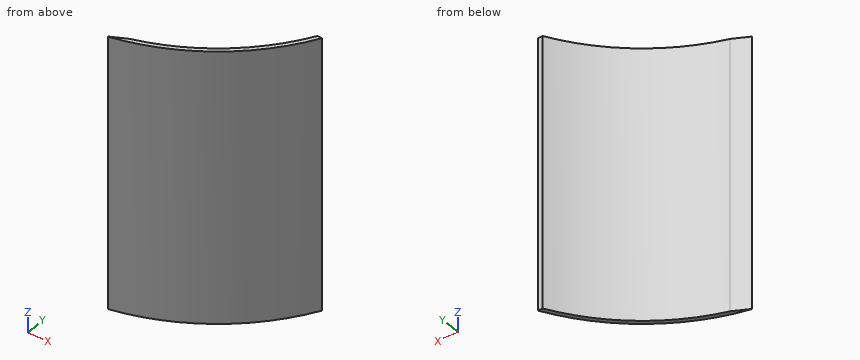
```python
from build123d import *

# Parameters (mm, degrees)
BOSS_EXTRUDE1_DEPTH = 200
CHAMFER1_SIZE       = 2.917865617


with BuildPart() as part:
    # Sketch1 → Boss-Extrude1 (new body)
    with BuildSketch(Plane.XY):
        with BuildLine():
            Line((100, 75), (96.575796241, 75))
            ThreePointArc((96.575796241, 75), (55.991051333, 28.692941942), (0, 3.071323807))
            Line((0, 3.071323807), (0, 0))
            ThreePointArc((0, 0), (58.18465914, 26.587121146), (100, 75))
        make_face()
    extrude(amount=BOSS_EXTRUDE1_DEPTH)

    # Chamfer1
    # the kernel refuses this chamfer: 10, 2.917865617 mm, written as the material it takes off along each edge
    with BuildSketch(Plane(origin=(0, 3.071323807, -30.394078092), x_dir=(0.9668531761663356, 0.25533298991134823, 0), z_dir=(0, 0, 1))) as chamfer1_piece_1:
        with BuildLine():
            Line((11.767108546, 0), (-CHAMFER1_SIZE * 0.255332989918, -CHAMFER1_SIZE * 0.96685317619))
            Line((-CHAMFER1_SIZE * 0.255332989918, -CHAMFER1_SIZE * 0.96685317619), (0, 0))
            ThreePointArc((0, 0), (6.078871228, -0.117659648), (11.767108546, 0))
        make_face()
    extrude(amount=260.788156184, mode=Mode.SUBTRACT)


solid = part.part
```
The model under review builds one solid part; all positions refer to its coordinate system, in mm. Round coordinates to 2 decimals unless told otherwise and drop trailing zeros. Order: outer loops, then holes, each group sorted by start corner. A loop starts at its lowest first (then second) coordinate and runs counter-clockwise, first axis right, second up. Notation, with made-up numbers: (61, 37) -> (76, 37) arc R23 cw to (76, 64) -> close; hole circle Ø3 at (-31, 41.25). An arc over 180 degrees is marked (long way). One line per item, written item: value. Start each with the question number.
Q1. Take a section at C-C (y = 40.5). Write out the cut boundary in (x, z), and give its area (3 significant figures).
Q2. Clearance check with flat-ended pins moving along their axes: pin 1 Ø5 at (x, z) = (37.5, 161.5) entering from -Y; pin 2 Ø2 at (x, z) = (48, 165.5) entering from +Y; pin 3 Ø8 at (y, z) = (34, 119.5) entering from -X. State where each tip first meets the part, or that it passes through.
Q3. Take a section at A-A (z = 33). Write out the cut boundary in (x, y), and give its area (3 significant figures).
Q4. Wall thickness on line 1 (Y direction, x = 31.5, z = 121); line 2 (X direction, y = 49, z = 29.5); line 3 (Y direction, x = 87, z = 149.5): over which ranges is each line inside the solid? List them lowest first.
Reported:
1. outline: (69.94, 0) -> (74.23, 0) -> (74.23, 200) -> (69.94, 200) -> close
1. area: 858 mm2
2. pin 1: stops at y = 12.29
2. pin 2: stops at y = 23.8
2. pin 3: stops at x = 57.72
3. outline: (0, 0) arc R150 ccw to (100, 75) -> (96.58, 75) arc R147 cw to (11.38, 6.08) -> (0, 0.15) -> close
3. area: 364 mm2
4. line 1: y = 10.6 to 13.92
4. line 2: x = 78.12 to 82.1
4. line 3: y = 55.03 to 60.03
